The model under review builds one solid part; all positions refer to its coordinate system, in mm. A direction names the side the tool comes from. Coordinates: 2 decimals unless noted, no trailing zeros. Order: outer loops, then holes, each group sorted by start corner. A loop starts at its lowest first (then second) coordinate and runs counter-clockwise, first axis right, second up. Notation, with made-up numbers: M 74,-21.5 L 103,-21.5 A37 ccw 103,17.5 Z; hole C -35.5,18.5 d4. An arc over 180 degrees is marked long. One line per item, written item: value.
```python
from build123d import *

# Parameters (mm, degrees)
BOSS_EXTRUDE1_DEPTH = 0.5
SKETCH2_R           = 1.4
BOSS_EXTRUDE2_DEPTH = 1.5
SKETCH3_R           = 1.4
BOSS_EXTRUDE3_DEPTH = 0.5
BOSS_EXTRUDE3_TAPER = 30


with BuildPart() as part:
    # Sketch1 → Boss-Extrude1 (new body)
    with BuildSketch(Plane.XY):
        Polygon((0, 3), (-2.598076211, 1.5), (-2.598076211, -1.5), (0, -3), (2.598076211, -1.5), (2.598076211, 1.5), align=None)
    extrude(amount=BOSS_EXTRUDE1_DEPTH)

    # Sketch2 → Boss-Extrude2 (add)
    with BuildSketch(Plane.XY.offset(0.5)):
        Circle(SKETCH2_R)
    extrude(amount=BOSS_EXTRUDE2_DEPTH)

    # Sketch3 → Boss-Extrude3 (add)
    with BuildSketch(Plane.XY.offset(2)):
        Circle(SKETCH3_R)
    extrude(amount=BOSS_EXTRUDE3_DEPTH, taper=BOSS_EXTRUDE3_TAPER)


solid = part.part
```
(1) We need section B-B, the plane z = 0.3. State the section outline as (x, y) points.
Geometry results:
outline: M -2.6,-1.5 L 0,-3 L 2.6,-1.5 L 2.6,1.5 L 0,3 L -2.6,1.5 Z
(2) We need section C-C, the plane z = 1.7. State the section outline as (x, y) points.
Geometry results:
outline: C 0,0 d2.8
(3) We need section A-A, the plane y = 0. State the section outline as (x, z) points.
Geometry results:
outline: M -2.6,0 L 2.6,0 L 2.6,0.5 L 1.4,0.5 L 1.4,2 L 1.11,2.5 L -1.11,2.5 L -1.4,2 L -1.4,0.5 L -2.6,0.5 Z
(4) We need section D-D, the plane x = -1.9. State the section outline as (y, z) points, plus the area to 3 significant figures.
Geometry results:
outline: M -1.9,0 L 1.9,0 L 1.9,0.5 L -1.9,0.5 Z
area: 1.90 mm2
(5) Tool access review of faces 1 (the flat face through (1.1, -1.3, 0.5)), 2 (the flat face through (-1.28, 2.26, 0.25)): name each direction out of +Z, -Z, +X, -X, +Y, -Y from which nothing blocks a thin tool from reaching the whole face with its end or side.
Geometry results:
face 1: +Z
face 2: +Z, -Z, -X, +Y
(6) For L1, parallel to Z at x = -1.2, y = 1.8; L2, parallel to Y at x = 0.75, z = 2.1; L3, parallel to X at y = -2.3, z = 0.35, list the stretches that pass through material, from the lowest coordinate up.
Geometry results:
L1: z = 0 to 0.5
L2: y = -1.11 to 1.11
L3: x = -1.21 to 1.21
